Read the model definition and answer for the solid it produces. Units are mm, in the model's axes. A direction names the side the tool comes from. Give positions to 0.01 mm unless a question says otherwise; leave off trailing zeros. Order: outer loops, then holes, each group sorted by start corner. A loop starts at its lowest first (then second) coordinate and runs counter-clockwise, first axis right, second up.
Item 1: A cutting plane is placed at D-D (z = -10.5). Write down the section's boundary in (x, y).
Item 2: The mould has two halves that part along Z. Classify faces 4 (the face through (34, -32, -42.535)), 5 (the face through (13, 17, 8.265)), 6 (the face through (34, -31, 20.965)), 7 (the face through (44, -52.876, -10)): +Z half, -Z half, draft (parallel to the pull), parting line (faces both ways), or undercut.
Item 3: Which of the six approach directions +Z, -Z, +X, -X, +Y, -Y give full straight-line access (tool end or side, diameter ignored) to faces 1 (the face through (70, -40, -4.435)), 2 (the face through (13, 10.624, -11)), 3 (the face through (50, -27.476, -11))?
Item 4: Find the intervals of material crossed by line 1 along Z through (x, y) = (66, -47); line 2 along X through (y, z) = (-27, -26); line 3 along Y through (x, z) = (61, 10), in increasing order.
Item 5: A cutting plane is placed at C-C (y = -30). Write down the section's boundary in (x, z).
Item 6: A cutting plane is placed at B-B (x = 12.5). Write down the section's boundary in (y, z), plus the area to 3 significant figures.
Item 7: A cutting plane is placed at A-A (x = 77). Write down the section's boundary in (y, z), plus the area to 3 significant figures.
Item 8: Given pin 1 Ø7.5 at (x, z) = (14, -1.5) entering from +Y; pin 2 Ø6.5 at (y, z) = (-37.5, -9.5) entering from +X; pin 3 Ø1.5 at (y, z) = (8.5, -32) entering from +X, each flat-ended and moving along its own axis, determine where each tip first touches the part or whether it passes through.
Autodesk Inventor part; units mm, degrees
ref_plane "YZ Plane" through (0, 0, 0) normal (1, 0, 0) x (0, 1, 0)
ref_plane "XZ Plane" through (0, 0, 0) normal (0, 1, 0) x (-1, 0, 0)
ref_plane "XY Plane" through (0, 0, 0) normal (0, 0, 1) x (1, 0, 0)
sketch "Sketch1" plane through (0, 0, 0) normal (1, 0, 0) x (0, 1, 0)
  line L0 (10.6243, 20.9647) -> (-52.8757, 20.9647)
  line L1 (-52.8757, 20.9647) -> (-52.8757, -42.5353)
  line L2 (-52.8757, -42.5353) -> (10.6243, -42.5353)
  line L3 (10.6243, -42.5353) -> (10.6243, 20.9647)
  point P0 (0, 0)
  dimension "d0" = 63.5
  dimension "d1" = 63.5
extrude "Extrusion1" add sketch "Sketch1" along normal blind 25.4
sketch "Sketch2" plane through (25.4, 0, 0) normal (1, 0, 0) x (0, 0, -1)
  line L0 (42.5353, 10.6243) -> (-20.9647, 10.6243)
  line L1 (-20.9647, 10.6243) -> (-8.2647, 10.6243)
  line L2 (-8.2647, 10.6243) -> (-8.2647, 23.3243)
  line L3 (-8.2647, 23.3243) -> (-20.9647, 23.3243)
  line L4 (-20.9647, 23.3243) -> (-20.9647, 10.6243)
  line L5 (42.5353, -52.8757) -> (42.5353, 10.6243)
  line L6 (42.5353, 10.6243) -> (29.8353, 10.6243)
  line L7 (29.8353, 10.6243) -> (29.8353, 23.3243)
  line L8 (29.8353, 23.3243) -> (42.5353, 23.3243)
  line L9 (42.5353, 23.3243) -> (42.5353, 10.6243)
  point P0 (0, 0)
  dimension "d4" = 12.7
  dimension "d5" = 12.7
  dimension "d6" = 12.7
  dimension "d7" = 12.7
extrude "Extrusion2" add sketch "Sketch2" against normal blind 25.4
sketch "Sketch3" plane through (25.4, 0, 0) normal (1, 0, 0) x (0, 0, -1)
  line L0 (-20.9647, -52.8757) -> (42.5353, -52.8757)
  line L1 (42.5353, -52.8757) -> (42.5353, -27.4757)
  line L2 (42.5353, -27.4757) -> (-20.9647, -27.4757)
  line L3 (-20.9647, -27.4757) -> (-20.9647, -52.8757)
  point P0 (0, 0)
  dimension "d10" = 63.5
  dimension "d11" = 25.4
extrude "Extrusion3" add sketch "Sketch3" along normal blind 63.5
sketch "Sketch4" plane through (88.9, 0, 0) normal (1, 0, 0) x (0, 0, -1)
  line L0 (-20.9647, 23.3243) -> (-20.9647, -52.8757)
  line L1 (-20.9647, -52.8757) -> (4.4353, -52.8757)
  line L2 (-20.9647, -52.8757) -> (42.5353, -52.8757)
  line L3 (4.4353, -52.8757) -> (4.4353, -27.4757)
  line L4 (42.5353, -27.4757) -> (-20.9647, -27.4757)
  line L5 (42.5353, -52.8757) -> (42.5353, -27.4757)
  line L6 (42.5353, -52.8757) -> (17.1353, -52.8757)
  line L7 (17.1353, -52.8757) -> (17.1353, -27.4757)
  line L8 (4.4353, -27.4757) -> (17.1353, -27.4757)
  line L9 (17.1353, -27.4757) -> (17.1353, -52.8757)
  line L10 (17.1353, -52.8757) -> (4.4353, -52.8757)
  line L11 (4.4353, -52.8757) -> (4.4353, -27.4757)
  point P0 (0, 0)
  dimension "d14" = 25.4
  dimension "d15" = 25.4
extrude "Extrusion4" cut sketch "Sketch4" against normal blind 38.1 contours L4 L7 L2 L3
properties part number "4.1e P3"
Response values:
1. outline: (0, -52.88) - (50.8, -52.88) - (50.8, -27.48) - (25.4, -27.48) - (25.4, 10.62) - (0, 10.62) - close
2. face 4: -Z half
2. face 5: undercut
2. face 6: +Z half
2. face 7: draft
3. face 1: +X, +Y, -Y
3. face 2: +X, -X, +Y
3. face 3: +Z, -Z, +X, +Y
4. line 1: z = -42.54 to -17.14, -4.44 to 20.96
4. line 2: x = 0 to 25.4
4. line 3: y = -52.88 to -27.48
5. outline: (0, -42.54) - (88.9, -42.54) - (88.9, -17.14) - (50.8, -17.14) - (50.8, -4.44) - (88.9, -4.44) - (88.9, 20.96) - (0, 20.96) - close
6. outline: (-52.88, -42.54) - (23.32, -42.54) - (23.32, -29.84) - (10.62, -29.84) - (10.62, 8.26) - (23.32, 8.26) - (23.32, 20.96) - (-52.88, 20.96) - close
6. area: 4,350 mm2
7. outline: (-52.88, -42.54) - (-27.48, -42.54) - (-27.48, -17.14) - (-52.88, -17.14) - close; (-52.88, -4.44) - (-27.48, -4.44) - (-27.48, 20.96) - (-52.88, 20.96) - close
7. area: 1,290 mm2
8. pin 1: stops at y = 10.62
8. pin 2: stops at x = 50.8
8. pin 3: stops at x = 25.4
